Verification items for this drawing (mm, ordinates from the low corner). Round coordinates to 2 decimals unless told otherwise and drop trailing zeros. Loops run counter-clockwise (first coordinate to the right, second up) from the corner with the lowest first, then second, coordinate; pieces in that order, holes last. Notation, with made-up numbers: M 59.25,-35.75 L 88.25,-35.75 A12 ccw 88.25,-12.75 Z; hole C 38.5,37.5 d7. An arc over 180 degrees is marked long. Use one line per item in the form item = value. Start each with the question number.
1. Cross-section at C-C (x = 125.5). Record the boundary of the cut face in (y, z).
2. Cross-section at A-A (x = 103.5). Record the boundary of the cut face in (y, z).
3. Go/stop test with flat-tipped pins: pin 1 (4.5 mm diameter, centred on x = 6.5, z = 90.36, fed in from +Y); pin 2 (12 mm diameter, centred on x = 86.5, z = 40.5, fed in from -Y). Record where each tip stops, or that it passes through.
4. Material ranges on line 1 (X direction, y = 3.8, z = 90.36); line 2 (Z direction, x = 37.5, y = 3.15); line 3 (Z direction, x = 125.5, y = 1.6), recorded low to high.
5. Cross-section at D-D (z = 90.36). Record the boundary of the cut face in (x, y), then the cut area to 3 significant figures.
6. Cross-section at B-B (z = 15.28). Record the boundary of the cut face in (x, y).
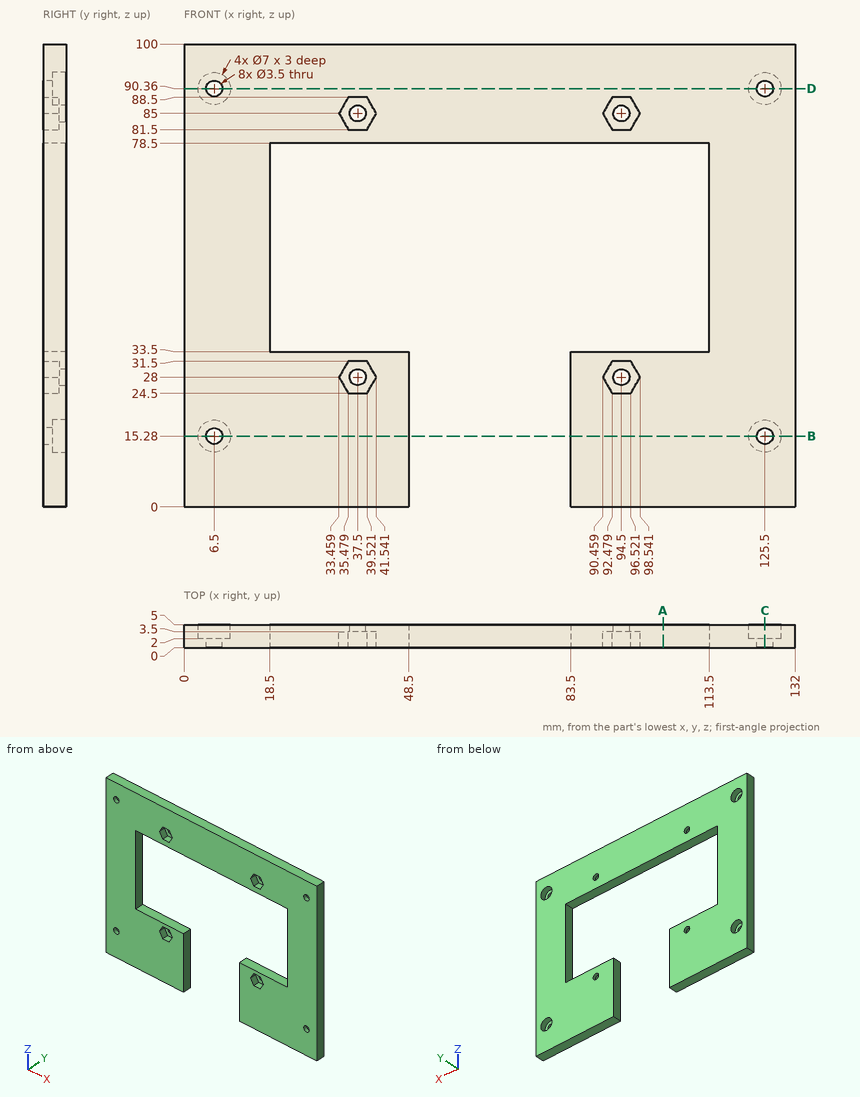
Reported:
q1.outline = M 0,0 L 5,0 L 5,11.78 L 2,11.78 L 2,13.53 L 0,13.53 Z; M 0,17.03 L 2,17.03 L 2,18.78 L 5,18.78 L 5,86.86 L 2,86.86 L 2,88.61 L 0,88.61 Z; M 0,92.11 L 2,92.11 L 2,93.86 L 5,93.86 L 5,100 L 0,100 Z
q2.outline = M 0,0 L 5,0 L 5,33.5 L 0,33.5 Z; M 0,78.5 L 5,78.5 L 5,100 L 0,100 Z
q3.pin_1 = 2
q3.pin_2 = through
q4.line_1 = 0 to 3, 10 to 122, 129 to 132
q4.line_2 = 0 to 24.5, 31.5 to 33.5, 78.5 to 81.5, 88.5 to 100
q4.line_3 = 0 to 13.53, 17.03 to 88.61, 92.11 to 100
q5.outline = M 0,0 L 4.75,0 L 4.75,2 L 3,2 L 3,5 L 0,5 Z; M 8.25,0 L 123.75,0 L 123.75,2 L 122,2 L 122,5 L 10,5 L 10,2 L 8.25,2 Z; M 127.25,0 L 132,0 L 132,5 L 129,5 L 129,2 L 127.25,2 Z
q5.area = 604 mm²
q6.outline = M 0,0 L 4.75,0 L 4.75,2 L 3,2 L 3,5 L 0,5 Z; M 8.25,0 L 48.5,0 L 48.5,5 L 10,5 L 10,2 L 8.25,2 Z; M 83.5,0 L 123.75,0 L 123.75,2 L 122,2 L 122,5 L 83.5,5 Z; M 127.25,0 L 132,0 L 132,5 L 129,5 L 129,2 L 127.25,2 Z
